Input: dimensioned drawing with shaded views. Units: mm. Origin: part minimum x, y, z. A direction names the side the tool comes from. Round coordinates to 2 decimals unless told otherwise and drop trailing zeros. Order: outer loops, then holes, each group sorted by start corner. A loop starts at its lowest first (then second) coordinate and runs counter-clockwise, first axis right, second up. Notation, with made-up numbers: M 61.25,-7 L 106.25,-7 A14 ccw 106.25,20 Z; hole C 84,17.25 d9. An arc over 180 degrees is marked long. Answer as CSV lines item,"result". Start each with the question number.
Item 1: Section query D-D on z = 2. Return the cut outline in (x, y), plus the area to 3 significant figures.
Item 2: Set-up query: the marked faces 3 and 4. Return all of +Z, -Z, +X, -X, +Y, -Y with unobstructed straight access to the full face (end or side cutting, diameter ignored); none if empty.
Item 3: Pull-direction query (X, two-part tool) for the marked faces 1 and 2; classes: +X half, -X half, draft (parallel to the pull), parting line (faces both ways), or undercut.
Item 4: Section query A-A on y = 3. Return the cut outline in (x, z), plus the area to 3 significant figures.
Item 5: Section query C-C on z = 9.75. Return the cut outline in (x, y), plus the area to 3 significant figures.
Item 6: First-contact query: P1, Ø1.5, axis at y = 2.5, z = 8.5, coming from the +X side; P2, Ø1, axis at y = 1.5, z = 22.5, coming from the +X side. Flat tips, straight axial feed; report the tip coordinate or a pass-through.
Item 7: Line query: line 1 (X direction, y = 3, z = 20); line 2 (Z direction, x = 1.15, y = 3); line 3 (X direction, y = 2.05, z = 14.5). Output: solid intervals per line, ascending. Write a range as [from, to].
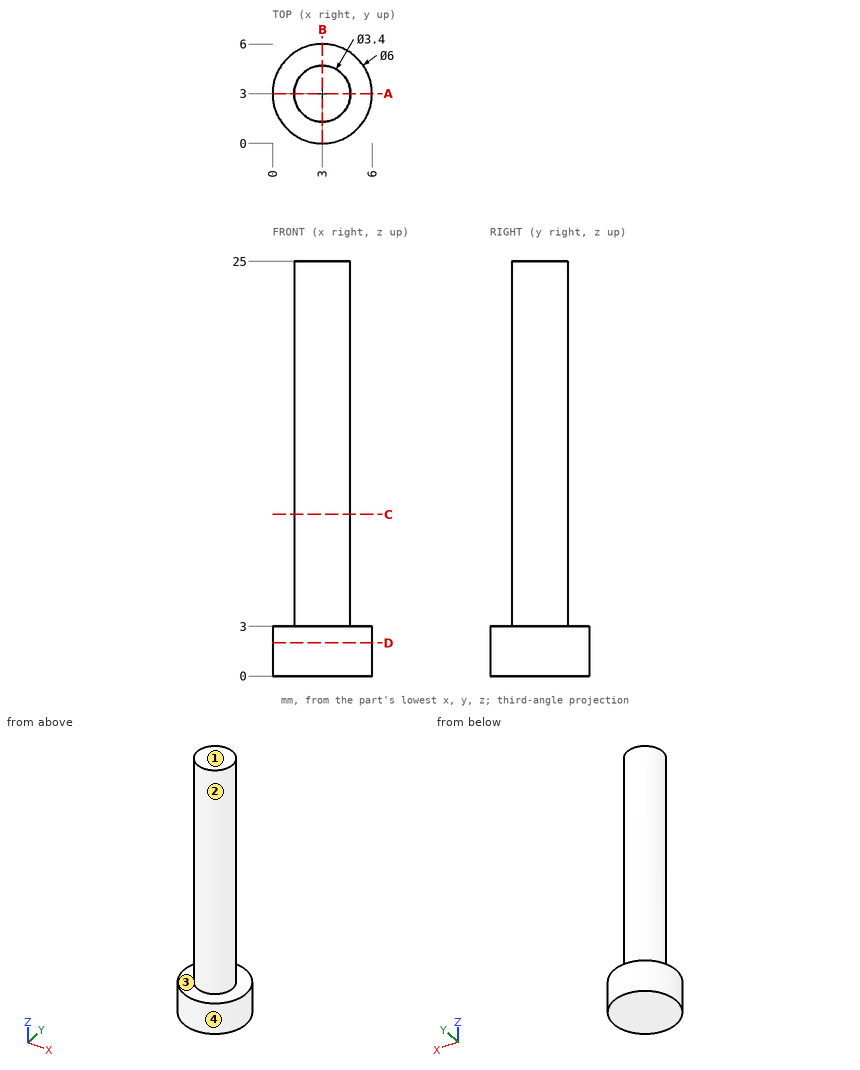
Results:
1,outline,"C 3,3 d6"
1,area,"28.3 mm^2"
2,face 3,"+Z"
2,face 4,"+Z, -Z"
3,face 1,"draft"
3,face 2,"parting line"
4,outline,"M 0,0 L 6,0 L 6,3 L 4.7,3 L 4.7,25 L 1.3,25 L 1.3,3 L 0,3 Z"
4,area,"92.8 mm^2"
5,outline,"C 3,3 d3.4"
5,area,"9.08 mm^2"
6,P1,"x = 4.7"
6,P2,"x = 4.37"
7,line 1,"[1.3, 4.7]"
7,line 2,"[0, 3]"
7,line 3,"[1.59, 4.41]"
